For this review, use the dimensioned drawing (mm, ordinates from the lowest corner) and the shaded views. Coordinates: 2 decimals unless noted, no trailing zeros. Order: outer loops, then holes, each group sorted by start corner. A loop starts at its lowest first (then second) coordinate and runs counter-clockwise, first axis right, second up. Notation, with made-up numbers: M 77,88 L 92,88 A21 ccw 92,105 Z; hole C 43,78.25 d9. An arc over 180 degrees is marked long. Use CSV: the item, a comma, the result in double quotes.
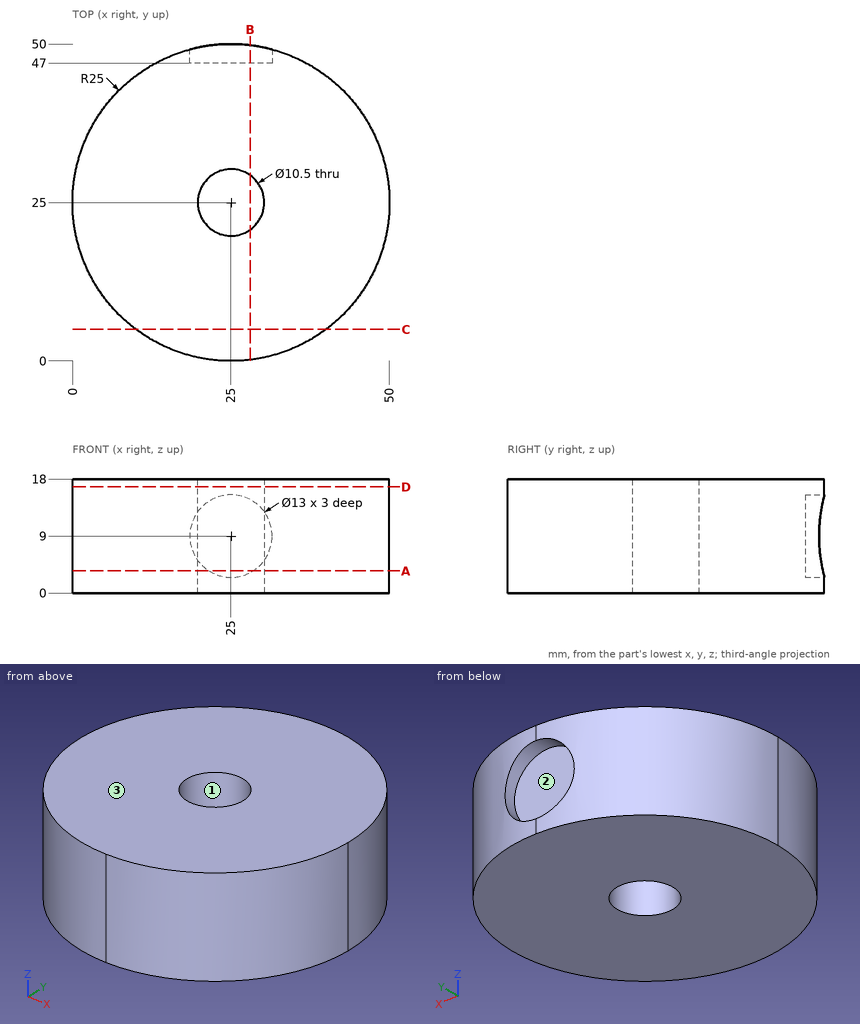
Item 1: Add section C-C on y = 5. State the section outline as (x, z) points.
Solutions:
outline,"M 10,0 L 40,0 L 40,18 L 10,18 Z"
Item 2: Add section A-A on z = 3.5. State the section outline as (x, y) points.
Solutions:
outline,"M 21.54,47 L 21.54,49.76 A25 ccw long 28.46,49.76 L 28.46,47 Z; hole C 25,25 d10.5"
Item 3: Add section D-D on z = 16.75. State the section outline as (x, y) points.
Solutions:
outline,"C 25,25 d50; hole C 25,25 d10.5"
Item 4: To check wall thickness, follow line 1 along X through (y, z) = (20.5, 1.75); line 2 along Y through (x, z) = (22, 12.75); line 3 along X through (y, z) = (48, 4.5). State the ranges of each line that lie inside material, in increasing order. Write a range as [from, to].
Solutions:
line 1,"[0.41, 22.3], [27.7, 49.59]"
line 2,"[0.18, 20.69], [29.31, 47]"
line 3,"[15.2, 20.31], [29.69, 34.8]"
Item 5: Add section B-B on x = 28. State the section outline as (y, z) points.
Solutions:
outline,"M 0.18,0 L 20.69,0 L 20.69,18 L 0.18,18 Z; M 29.31,0 L 49.82,0 L 49.82,3.23 L 47,3.23 L 47,14.77 L 49.82,14.77 L 49.82,18 L 29.31,18 Z"
Item 6: Draft analysis for pull direction Z (two halves, no side actions). For the marked faces 1, 2 and 3, state which applies: released by +Z, released by -Z, zero draft, split by the parting line, or undercut.
Solutions:
face 1,"zero draft"
face 2,"undercut"
face 3,"released by +Z"
Item 7: Clearance check with flat-ended pins moving along their axes: pin 1 Ø3 at (y, z) = (28, 9) entering from +X; pin 2 Ø10.5 at (x, z) = (25, 9) entering from +Y; pin 3 Ø10 at (x, z) = (12, 10.5) entering from -Y. State where each tip first meets the part, or that it passes through.
Solutions:
pin 1,"x = 49.95"
pin 2,"y = 47"
pin 3,"y = 1.31"
